For this review, take the finished solid that the model builds, in its own axes (mm). Coordinates: 2 decimals unless noted, no trailing zeros. Write each loop counter-clockwise with the first axis right and the second up, starting at its lowest first coordinate (ties: lowest second). Pieces come first, ordered by that corner, then holes. Notation, with made-up numbers: M -6,-39 L 41,-39 A14 ccw 41,-12 Z; hole C -32.5,87 d11. An arc over 180 degrees is marked long. One line per question, with ' | ' between items.
from build123d import *

# Parameters (mm, degrees)
F1_DEPTH     = 22.5
F2_R         = 18.6
F3_DEPTH     = 6
F4_R         = 17.5
F5_DEPTH     = 3
F7_DEPTH     = 3
F8_DEPTH     = 3
F14_DEPTH    = 3
F9_T1_DEPTH  = 3
F9_T6_DEPTH  = 3
F9_T11_DEPTH = 3
F15_W        = 6
F15_H        = 97.4
F10_DEPTH    = 45.001
F11_R        = 1.49999


# Not quite as in the source:
# - a fillet or chamfer that OpenCascade refuses, or shapes differently, is made with other operations: its cross-section is extruded or revolved along the edge and cut away or added
# - a fillet or chamfer is up to 0.001 mm smaller than in the source, because OpenCascade refuses the exact size


with BuildPart() as f1:
    # F0 (on Right) → F1 (new body, symmetric)
    with BuildSketch(Plane.YZ):
        Polygon((0, -25), (0, 25), (-3, 25), (-3, 21.25), (-9, 21.25), (-9, -21.25), (-3, -21.25), (-3, -25), align=None)
    extrude(amount=F1_DEPTH, both=True)

    # F2 (on face) → F3 (cut)
    with BuildSketch(Plane.XZ.offset(9)):
        Circle(F2_R)
    extrude(amount=-F3_DEPTH, mode=Mode.SUBTRACT)

    # F4 (on face) → F5 (cut, through all)
    with BuildSketch(Plane.XZ.offset(3)):
        Circle(F4_R)
    extrude(amount=-F5_DEPTH, mode=Mode.SUBTRACT)

    # F6 (on face) → F7 (join)
    with BuildSketch(Plane.XZ.offset(9)):
        with BuildLine():
            Line((-1.6773361726, 21.1145450883), (-1.5, 21.05))
            Line((-1.5, 21.05), (2.8857066002, 21.05))
            Line((2.8857066002, 21.05), (-1.1643059576, 22.5240840195))
            ThreePointArc((-1.1643059576, 22.5240840195), (-1.8221335094, 23.4812290467), (-1.1313028087, 24.4148331565))
            Line((-1.1313028087, 24.4148331565), (1.1823725422, 25.1665918487))
            ThreePointArc((1.1823725422, 25.1665918487), (2.9098300563, 27.5442331395), (1.1823725422, 29.9218744302))
            Line((1.1823725422, 29.9218744302), (-2.6423503277, 31.1646022233))
            ThreePointArc((-2.6423503277, 31.1646022233), (-3.3282367753, 32.0148264964), (-2.8268835217, 32.9853760566))
            Line((-2.8268835217, 32.9853760566), (3.5672088043, 36.6139176646))
            ThreePointArc((3.5672088043, 36.6139176646), (4.8205919381, 39.0402915651), (3.1058758193, 41.165852248))
            Line((3.1058758193, 41.165852248), (-0.0769036922, 42.2))
            Line((-0.0769036922, 42.2), (-4.9310056584, 42.2))
            Line((-4.9310056584, 42.2), (2.6423503277, 39.7392674735))
            ThreePointArc((2.6423503277, 39.7392674735), (3.3282367753, 38.8890432004), (2.8268835217, 37.9184936402))
            Line((2.8268835217, 37.9184936402), (-3.5672088043, 34.2899520321))
            ThreePointArc((-3.5672088043, 34.2899520321), (-4.8205919381, 31.8635781317), (-3.1058758193, 29.7380174488))
            Line((-3.1058758193, 29.7380174488), (0.7188470506, 28.4952896558))
            ThreePointArc((0.7188470506, 28.4952896558), (1.4098300563, 27.5442331395), (0.7188470506, 26.5931766232))
            Line((0.7188470506, 26.5931766232), (-1.5948283002, 25.841417931))
            ThreePointArc((-1.5948283002, 25.841417931), (-3.3219050522, 23.5074076563), (-1.6773361726, 21.1145450883))
        make_face()
        with BuildLine():
            Line((3.5672088043, -36.6139176646), (-2.8268835217, -32.9853760566))
            ThreePointArc((-2.8268835217, -32.9853760566), (-3.3282367753, -32.0148264964), (-2.6423503277, -31.1646022233))
            Line((-2.6423503277, -31.1646022233), (1.1823725422, -29.9218744302))
            ThreePointArc((1.1823725422, -29.9218744302), (2.9098300563, -27.5442331395), (1.1823725422, -25.1665918487))
            Line((1.1823725422, -25.1665918487), (-1.1313028087, -24.4148331565))
            ThreePointArc((-1.1313028087, -24.4148331565), (-1.8221335094, -23.4812290467), (-1.1643059576, -22.5240840195))
            Line((-1.1643059576, -22.5240840195), (2.8857066002, -21.05))
            Line((2.8857066002, -21.05), (-1.5, -21.05))
            Line((-1.5, -21.05), (-1.6773361726, -21.1145450883))
            ThreePointArc((-1.6773361726, -21.1145450883), (-3.3219050522, -23.5074076563), (-1.5948283002, -25.841417931))
            Line((-1.5948283002, -25.841417931), (0.7188470506, -26.5931766232))
            ThreePointArc((0.7188470506, -26.5931766232), (1.4098300563, -27.5442331395), (0.7188470506, -28.4952896558))
            Line((0.7188470506, -28.4952896558), (-3.1058758193, -29.7380174488))
            ThreePointArc((-3.1058758193, -29.7380174488), (-4.8205919381, -31.8635781317), (-3.5672088043, -34.2899520321))
            Line((-3.5672088043, -34.2899520321), (2.8268835217, -37.9184936402))
            ThreePointArc((2.8268835217, -37.9184936402), (3.3282367753, -38.8890432004), (2.6423503277, -39.7392674735))
            Line((2.6423503277, -39.7392674735), (-4.9310056584, -42.2))
            Line((-4.9310056584, -42.2), (-0.0769036922, -42.2))
            Line((-0.0769036922, -42.2), (3.1058758193, -41.165852248))
            ThreePointArc((3.1058758193, -41.165852248), (4.8205919381, -39.0402915651), (3.5672088043, -36.6139176646))
        make_face()
    extrude(amount=-F7_DEPTH)

    # F12 (on face) → F8 (join)
    with BuildSketch(Plane.XZ.offset(9)):
        with BuildLine():
            Line((-10.0039546753, 45.1082380117), (-10.0039546753, 41.7))
            Line((-10.0039546753, 41.7), (-2.5039546753, 41.7))
            Line((-2.5039546753, 41.7), (4.9960453247, 41.7))
            Line((4.9960453247, 41.7), (4.9960453247, 45.1082380117))
            ThreePointArc((4.9960453247, 45.1082380117), (4.9619908828, 45.2896070742), (4.8644663773, 45.446270448))
            ThreePointArc((4.8644663773, 45.446270448), (-2.5039546753, 48.6856217223), (-9.872375728, 45.446270448))
            ThreePointArc((-9.872375728, 45.446270448), (-9.9699002335, 45.2896070742), (-10.0039546753, 45.1082380117))
        make_face()
        with BuildLine():
            Line((4.9960453247, -41.7), (-10.0039546753, -41.7))
            Line((-10.0039546753, -41.7), (-10.0039546753, -45.1082380117))
            ThreePointArc((-10.0039546753, -45.1082380117), (-9.9699002335, -45.2896070742), (-9.872375728, -45.446270448))
            ThreePointArc((-9.872375728, -45.446270448), (-2.5039546753, -48.6856217223), (4.8644663773, -45.446270448))
            ThreePointArc((4.8644663773, -45.446270448), (4.9619908828, -45.2896070742), (4.9960453247, -45.1082380117))
            Line((4.9960453247, -45.1082380117), (4.9960453247, -41.7))
        make_face()
    extrude(amount=-F8_DEPTH)

    # F13 (on face) → F14 (join)
    with BuildSketch(Plane(origin=(0, -6, 0), x_dir=(-1, 0, 0), z_dir=(0, 1, 0))):
        Polygon((-4.9960453247, 41.7), (10.0039546753, 41.7), (10.0039546753, 41.9), (9.0039546753, 42.9), (8.0039546753, 41.9), (7.0039546753, 42.9), (6.0039546753, 41.9), (5.0039546753, 42.9), (4.0039546753, 41.9), (3.0039546753, 42.9), (2.0039546753, 41.9), (1.0039546753, 42.9), (0.0039546753, 41.9), (-0.9960453247, 42.9), (-1.9960453247, 41.9), (-2.9960453247, 42.9), (-3.9960453247, 41.9), (-4.9960453247, 42.9), align=None)
        Polygon((-4.9960453247, -41.7), (-4.9960453247, -42.9), (-3.9960453247, -41.9), (-2.9960453247, -42.9), (-1.9960453247, -41.9), (-0.9960453247, -42.9), (0.0039546753, -41.9), (1.0039546753, -42.9), (2.0039546753, -41.9), (3.0039546753, -42.9), (4.0039546753, -41.9), (5.0039546753, -42.9), (6.0039546753, -41.9), (7.0039546753, -42.9), (8.0039546753, -41.9), (9.0039546753, -42.9), (10.0039546753, -41.9), (10.0039546753, -41.7), align=None)
    extrude(amount=F14_DEPTH)

    # F9: fillet of radius 1 on 8 edges, made by hand

    # F9_s2 → F9_t1 (join)
    with BuildSketch(Plane.XZ.offset(6)):
        with BuildLine():
            ThreePointArc((-3.1671397399, 22.5967933258), (-3.2844738139, 21.6785077979), (-4.1050813101, 21.25))
            Line((-4.1050813101, 21.25), (-1.9838334832, 21.25))
            ThreePointArc((-1.9838334832, 21.25), (-2.7003635819, 21.813678492), (-3.1671397399, 22.5967933258))
        make_face()
        with BuildLine():
            ThreePointArc((2.1705179537, 21.3103073792), (2.3388899194, 21.265192247), (2.5125380971, 21.25))
            Line((2.5125380971, 21.25), (2.3362111164, 21.25))
            Line((2.3362111164, 21.25), (2.1705179537, 21.3103073792))
        make_face()
        with BuildLine():
            ThreePointArc((-3.2415313358, 41.6510565163), (-3.3941138651, 41.6876883406), (-3.5505483302, 41.7))
            Line((-3.5505483302, 41.7), (-3.3921638899, 41.7))
            Line((-3.3921638899, 41.7), (-3.2415313358, 41.6510565163))
        make_face()
        with BuildLine():
            ThreePointArc((-3.1671397399, -22.5967933258), (-3.2844738139, -21.6785077979), (-4.1050813101, -21.25))
            Line((-4.1050813101, -21.25), (-1.9838334832, -21.25))
            ThreePointArc((-1.9838334832, -21.25), (-2.7003635819, -21.813678492), (-3.1671397399, -22.5967933258))
        make_face()
        with BuildLine():
            ThreePointArc((-3.5505483302, -41.7), (-3.3941138651, -41.6876883406), (-3.2415313358, -41.6510565163))
            Line((-3.2415313358, -41.6510565163), (-3.3921638899, -41.7))
            Line((-3.3921638899, -41.7), (-3.5505483302, -41.7))
        make_face()
        with BuildLine():
            ThreePointArc((2.1705179537, -21.3103073792), (2.3388899194, -21.265192247), (2.5125380971, -21.25))
            Line((2.5125380971, -21.25), (2.3362111164, -21.25))
            Line((2.3362111164, -21.25), (2.1705179537, -21.3103073792))
        make_face()
    extrude(amount=F9_T1_DEPTH)


with BuildPart() as f9_tool4:
    # F9_s5 → F9_t6 (new body)
    with BuildSketch(Plane.XZ.offset(9)):
        with BuildLine():
            ThreePointArc((5.265067062, 41.7), (4.3857987751, 41.1763268621), (4.4274288538, 40.1537745592))
            Line((4.4274288538, 40.1537745592), (4.343665033, 40.0991520151))
            ThreePointArc((4.343665033, 40.0991520151), (3.0749741198, 41.0707465963), (1.431036377, 41.6048943484))
            Line((1.431036377, 41.6048943484), (1.4619380764, 41.8))
            Line((1.4619380764, 41.8), (5.265067062, 41.8))
            Line((5.265067062, 41.8), (5.265067062, 41.7))
        make_face()
    extrude(amount=-F9_T6_DEPTH)

    split(bisect_by=Plane.YZ.offset(4.9960453247), keep=Keep.BOTTOM)


with BuildPart() as f1_1:
    add(f1.part)

    # F9_t3: union F9_tool4
    add(f9_tool4.part)


with BuildPart() as f9_tool9:
    # F9_s10 → F9_t11 (new body)
    with BuildSketch(Plane.XZ.offset(6)):
        with BuildLine():
            ThreePointArc((4.4274288538, -40.1537745592), (4.3857987751, -41.1763268621), (5.265067062, -41.7))
            Line((5.265067062, -41.7), (5.265067062, -41.8))
            Line((5.265067062, -41.8), (1.4619380764, -41.8))
            Line((1.4619380764, -41.8), (1.431036377, -41.6048943484))
            ThreePointArc((1.431036377, -41.6048943484), (3.0749741198, -41.0707465963), (4.343665033, -40.0991520151))
            Line((4.343665033, -40.0991520151), (4.4274288538, -40.1537745592))
        make_face()
    extrude(amount=F9_T11_DEPTH)

    split(bisect_by=Plane.YZ.offset(4.9960453247), keep=Keep.BOTTOM)


with BuildPart() as f1_2:
    add(f1_1.part)

    # F9_t8: union F9_tool9
    add(f9_tool9.part)

    # F15 (on face) → F10 (cut, through all)
    with BuildSketch(Plane.YZ.offset(22.5)):
        with Locations((-6, 0)):
            Rectangle(F15_W, F15_H)
    extrude(amount=-F10_DEPTH, mode=Mode.SUBTRACT)

    # F11 (radius 1.5 in the source; OpenCascade refuses exactly that, so slightly less here)
    f11_edges = [f1_2.edges().sort_by_distance(p)[0] for p in [
        (0, -3, 25),
        (0, 0, 25),
        (0, -3, -25),
        (0, 0, -25),
    ]]
    fillet(f11_edges, radius=F11_R)


solid = f1_2.part
1. Take a section at D-D on z = 13. State the section outline as (x, y) points, plus the area to 3 significant figures.
Computed values:
outline: M -22.5,-3 L -11.72,-3 L -11.72,0 L -22.5,0 Z; M 11.72,-3 L 22.5,-3 L 22.5,0 L 11.72,0 Z | area: 64.7 mm2
2. Take a section at B-B on z = 0. State the section outline as (x, y) points.
Computed values:
outline: M -22.5,-3 L -17.5,-3 L -17.5,0 L -22.5,0 Z; M 17.5,-3 L 22.5,-3 L 22.5,0 L 17.5,0 Z
3. Draft analysis for pull direction Z (two halves, no side actions). For faces 1 (the flat face through (-22.5, -2, 0)), 2 (the cylindrical face through (-0.32, -0.43, -24.55)), 3 (the cylindrical face through (-13.887, -1.521, -10.648)), state which applies: pulls with the +Z half, pulls with the -Z half, needs draft (parallel to the pull), parting line crosses it, or undercut.
Computed values:
face 1: needs draft | face 2: pulls with the -Z half | face 3: undercut
4. For line 1 along Z through (x, y) = (0, -1.5); line 2 along Z through (x, y) = (-12.5, -0.95); line 3 along X through (y, z) = (-2.65, -14.5), list the stretches that pass through material, from the lowest coordinate up.
Computed values:
line 1: z = -25 to -17.5, 17.5 to 25 | line 2: z = -24.9 to -12.25, 12.25 to 24.9 | line 3: x = -22.5 to -9.8, 9.8 to 22.5
5. Clearance check with a flat-ended pin moving along its axis: P1, Ø2, axis at x = -14.5, z = 6.5, coming from the +Y side. State where the tip first meets the part, or that it passes through.
Computed values:
P1: passes through
6. Take a section at C-C on y = -2.45. State the section outline as (x, z) points.
Computed values:
outline: M -22.5,-24.66 L 22.5,-24.66 L 22.5,24.66 L -22.5,24.66 Z; hole C 0,0 d35
